```python
from build123d import *

# Parameters (mm, degrees)
SKETCH1_R           = 2
SKETCH1_R_2         = 3.5
SKETCH1_R_3         = 16
BOSS_EXTRUDE1_DEPTH = 20
CUT_EXTRUDE1_DEPTH  = 2
CUT_EXTRUDE2_START  = -3
CUT_EXTRUDE2_DEPTH  = 2
LPATTERN1_COUNT     = 7
LPATTERN1_PITCH     = 5
SKETCH2_R           = 18
SKETCH2_R_2         = 16
CUT_EXTRUDE3_DEPTH  = 2


with BuildPart() as part:
    # Sketch1 → Boss-Extrude1 (new, symmetric)
    with BuildSketch(Plane(origin=(0, 0, 0), x_dir=(1, 0, 0), z_dir=(0, 1, 0))):
        with BuildLine():
            Line((-22, 22.5), (-24, 22.5))
            ThreePointArc((-24, 22.5), (-26.828427125, 21.328427125), (-28, 18.5))
            Line((-28, 18.5), (-28, -18.5))
            ThreePointArc((-28, -18.5), (-26.828427125, -21.328427125), (-24, -22.5))
            Line((-24, -22.5), (-22, -22.5))
            Line((-22, -22.5), (18, -22.5))
            ThreePointArc((18, -22.5), (20.828427125, -21.328427125), (22, -18.5))
            Line((22, -18.5), (22, 18.5))
            ThreePointArc((22, 18.5), (20.828427125, 21.328427125), (18, 22.5))
            Line((18, 22.5), (-22, 22.5))
        make_face()
        with Locations(Location((-24, 0, 0), (0, 0, 270))):
            Circle(SKETCH1_R, mode=Mode.SUBTRACT)
        with Locations(Location((16.079705534, 16.445153387, 0), (0, 0, 270))):
            Circle(SKETCH1_R_2, mode=Mode.SUBTRACT)
        with Locations(Location((-16.079705534, 16.445153387, 0), (0, 0, 270))):
            Circle(SKETCH1_R_2, mode=Mode.SUBTRACT)
        with Locations(Location((-16.079705534, -16.445153387, 0), (0, 0, 270))):
            Circle(SKETCH1_R_2, mode=Mode.SUBTRACT)
        with Locations(Location((16.079705534, -16.445153387, 0), (0, 0, 270))):
            Circle(SKETCH1_R_2, mode=Mode.SUBTRACT)
        with Locations(Location((0, 0, 0), (0, 0, 270))):
            Circle(SKETCH1_R_3, mode=Mode.SUBTRACT)
    extrude(amount=BOSS_EXTRUDE1_DEPTH, both=True)

    # Sketch3 → Cut-Extrude1 (cut)
    with BuildSketch(Plane(origin=(0, 20, 0), x_dir=(1, 0, 0), z_dir=(0, 1, 0))):
        with BuildLine():
            Line((-24, 2), (-15.874507866, 2))
            ThreePointArc((-15.874507866, 2), (-16, 0), (-15.874507866, -2))
            Line((-15.874507866, -2), (-24, -2))
            ThreePointArc((-24, -2), (-22, 0), (-24, 2))
        make_face()
    extrude(amount=-CUT_EXTRUDE1_DEPTH, mode=Mode.SUBTRACT)

    # Sketch5 → Cut-Extrude2 (cut)
    with BuildSketch(Plane(origin=(0, 20, 0), x_dir=(1, 0, 0), z_dir=(0, 1, 0)).offset(CUT_EXTRUDE2_START)):
        with BuildLine():
            ThreePointArc((13.266499161, -22.5), (6.92820323, -19.521749414), (0, -18.5))
            Line((0, -18.5), (0, -22.5))
            Line((0, -22.5), (13.266499161, -22.5))
        make_face()
        with BuildLine():
            Line((0, -22.5), (0, -18.5))
            ThreePointArc((0, -18.5), (-6.92820323, -19.521749414), (-13.266499161, -22.5))
            Line((-13.266499161, -22.5), (0, -22.5))
        make_face()
        with BuildLine():
            Line((13.266499161, -22.5), (0, -22.5))
            Line((0, -22.5), (-13.266499161, -22.5))
            ThreePointArc((-13.266499161, -22.5), (-11.349097324, -63.647056295), (24, -42.5))
            ThreePointArc((24, -42.5), (21.147056295, -31.150902676), (13.266499161, -22.5))
        make_face()
        with BuildLine():
            ThreePointArc((18, 0), (19.021749414, -6.92820323), (22, -13.266499161))
            Line((22, -13.266499161), (22, 0))
            Line((22, 0), (18, 0))
        make_face()
        with BuildLine():
            Line((22, 0), (22, -13.266499161))
            ThreePointArc((22, -13.266499161), (48.92820323, -22.978250586), (66, 0))
            ThreePointArc((66, 0), (48.92820323, 22.978250586), (22, 13.266499161))
            Line((22, 13.266499161), (22, 0))
        make_face()
        with BuildLine():
            Line((18, 0), (22, 0))
            Line((22, 0), (22, 13.266499161))
            ThreePointArc((22, 13.266499161), (19.021749414, 6.92820323), (18, 0))
        make_face()
        with BuildLine():
            ThreePointArc((24, 42.5), (-11.349097324, 63.647056295), (-13.266499161, 22.5))
            Line((-13.266499161, 22.5), (0, 22.5))
            Line((0, 22.5), (13.266499161, 22.5))
            ThreePointArc((13.266499161, 22.5), (21.147056295, 31.150902676), (24, 42.5))
        make_face()
        with BuildLine():
            Line((0, 22.5), (-13.266499161, 22.5))
            ThreePointArc((-13.266499161, 22.5), (-6.92820323, 19.521749414), (0, 18.5))
            Line((0, 18.5), (0, 22.5))
        make_face()
        with BuildLine():
            Line((13.266499161, 22.5), (0, 22.5))
            Line((0, 22.5), (0, 18.5))
            ThreePointArc((0, 18.5), (6.92820323, 19.521749414), (13.266499161, 22.5))
        make_face()
    cut_extrude2 = extrude(amount=-CUT_EXTRUDE2_DEPTH, mode=Mode.SUBTRACT)

    # LPattern1: Cut-Extrude2 ×7
    with Locations(*[(0, -i * LPATTERN1_PITCH, 0) for i in range(1, LPATTERN1_COUNT)]):
        add(cut_extrude2, mode=Mode.SUBTRACT)

    # Sketch2 → Cut-Extrude3 (cut)
    with BuildSketch(Plane.XZ.offset(20)):
        with Locations(Location((0, 0, 0), (0, 0, 270))):
            Circle(SKETCH2_R)
        with Locations(Location((0, 0, 0), (0, 0, 270))):
            Circle(SKETCH2_R_2, mode=Mode.SUBTRACT)
    extrude(amount=-CUT_EXTRUDE3_DEPTH, mode=Mode.SUBTRACT)


solid = part.part
```
Read the model definition and answer for the solid it produces. Units are mm, in the model's axes. A direction names the side the tool comes from. Give positions to 0.01 mm unless a question says otherwise; leave off trailing zeros. Loops run counter-clockwise (first coordinate to the right, second up) from the corner with the lowest first, then second, coordinate; pieces in that order, holes last.
Item 1: For faces 4 (the flat face through (0, -5, 21)), 5 (the cylindrical face through (12.663, -0.28, 15.686)), 6 (the flat face through (20, -15, 0)), 7 (the flat face through (0, 10, -21)), 8 (the flat face through (-20, -20, 0)), determine the directions among +Z, -Z, +X, -X, +Y, -Y from which every point of the face is accessible in a straight line to the end or side of a thin tool.
Item 2: The part is cut by section B-B (z = -14). Write down the section's boundary in (x, y).
Item 3: The mould has two halves that part along Z. Classify faces 1 (the flat face through (0, 17, -21)), 2 (the flat face through (20, -5, 0)), 3 (the flat face through (-3.3, 4.7, 22.5)): released by +Z, released by -Z, zero draft, split by the parting line, or undercut.
Item 4: This flat-tipped pin is pushed along its axis until it touches: pin 1 Ø2.5 at (x, z) = (-24, 0) entering from +Y (3 decimals). Where does it stop, or does it pass through?
Item 5: The part is cut by section C-C (y = 14). Write down the section's boundary in (x, z), and give its area (3 significant figures).
Item 6: Find the intervals of material crossed by line 1 along X through (y, z) = (-1, 0); line 2 along X through (y, z) = (8, -17.5); line 3 along Z through (x, y) = (18.5, -16), in increasing order.
Item 7: The part is cut by section A-A (x = -14). Write down the section's boundary in (y, z).
Taken from the geometry:
1. face 4: +Z
1. face 5: +Y, -Y
1. face 6: +X
1. face 7: -Z
1. face 8: +Z, -Z, +X, -X, -Y
2. outline: (-28, -20) - (-18.58, -20) - (-18.58, 20) - (-28, 20) - close; (-13.58, -20) - (-11.31, -20) - (-11.31, -18) - (-7.75, -18) - (-7.75, 20) - (-13.58, 20) - close; (7.75, -18) - (11.31, -18) - (11.31, -20) - (13.58, -20) - (13.58, 20) - (7.75, 20) - close; (18.58, -20) - (22, -20) - (22, 20) - (18.58, 20) - close
3. face 1: zero draft
3. face 2: undercut
3. face 3: released by +Z
4. pin 1: passes through
5. outline: (-28, -18.5) arc R4 ccw to (-24, -22.5) - (18, -22.5) arc R4 ccw to (22, -18.5) - (22, 18.5) arc R4 ccw to (18, 22.5) - (-24, 22.5) arc R4 ccw to (-28, 18.5) - close; hole circle Ø4 at (-24, 0); hole circle Ø7 at (-16.08, -16.45); hole circle Ø7 at (-16.08, 16.45); hole circle Ø32 at (0, 0); hole circle Ø7 at (16.08, -16.45); hole circle Ø7 at (16.08, 16.45)
5. area: 1,270 mm2
6. line 1: x = -28 to -26, -22 to -16, 16 to 22
6. line 2: x = -28 to -19.42, -12.74 to 12.74, 19.42 to 22
6. line 3: z = -22.47 to -18.97, -13.92 to 13.92, 18.97 to 22.47
7. outline: (-20, -22.5) - (20, -22.5) - (20, -19.26) - (-20, -19.26) - close; (-20, -13.63) - (20, -13.63) - (20, -7.75) - (-18, -7.75) - (-18, -11.31) - (-20, -11.31) - close; (-20, 11.31) - (-18, 11.31) - (-18, 7.75) - (20, 7.75) - (20, 13.63) - (-20, 13.63) - close; (-20, 19.26) - (20, 19.26) - (20, 22.5) - (-20, 22.5) - close
